Geometry check sheet. Reference: drawing and pictorial views, mm from the part's lowest x, y, z. Round coordinates to 2 decimals unless told otherwise and drop trailing zeros. Write each loop counter-clockwise with the first axis right and the second up, starting at its lowest first coordinate (ties: lowest second). Pieces come first, ordered by that corner, then holes. Notation, with made-up numbers: M -29,89 L 21,89 A13 cw 21,106 Z; hole C 32.5,72 d2. An arc over 180 degrees is marked long. One line per question, with ' | ' between items.
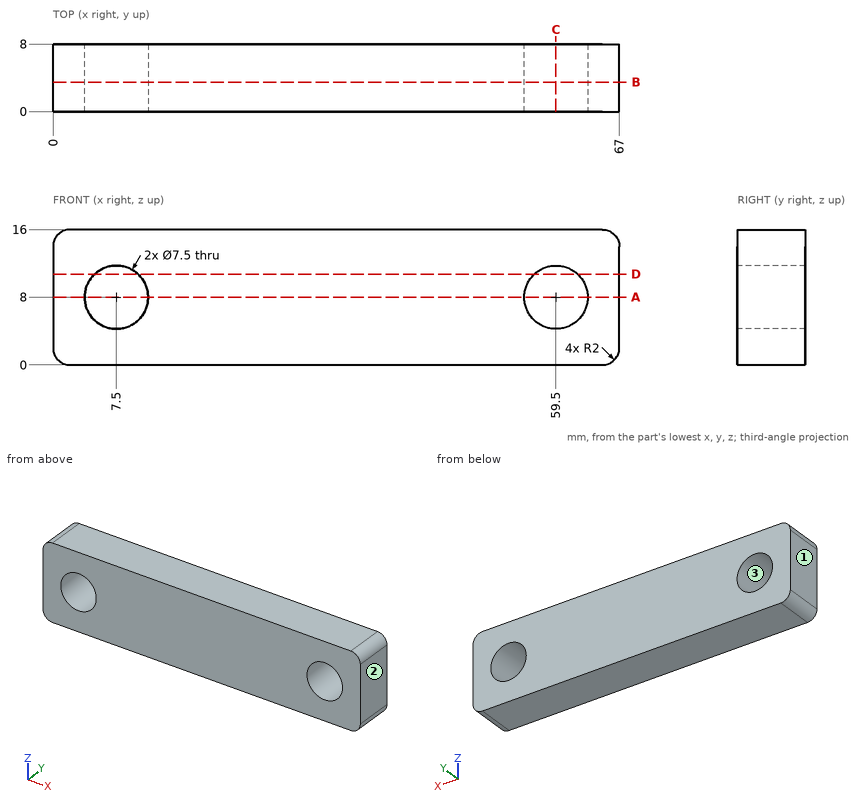
1. Section check C-C, the plane x = 59.5. Record the cut outline in (y, z).
Results:
outline: M 0,0 L 8,0 L 8,4.25 L 0,4.25 Z; M 0,11.75 L 8,11.75 L 8,16 L 0,16 Z
2. Section check D-D, the plane z = 10.75. Record the cut outline in (x, y), then the cut area to 3 significant figures.
Results:
outline: M 0,0 L 4.95,0 L 4.95,8 L 0,8 Z; M 10.05,0 L 56.95,0 L 56.95,8 L 10.05,8 Z; M 62.05,0 L 67,0 L 67,8 L 62.05,8 Z | area: 454 mm2
3. Section check B-B, the plane y = 3.5. Record the cut outline in (x, z).
Results:
outline: M 0,2 A2 ccw 2,0 L 65,0 A2 ccw 67,2 L 67,14 A2 ccw 65,16 L 2,16 A2 ccw 0,14 Z; hole C 7.5,8 d7.5; hole C 59.5,8 d7.5
4. Mould release check, pull along X, two halves, no side actions. Record for the marked faces 1, 2 and 3: pulls with the +X half, pulls with the -X half, needs draft (parallel to the pull), parting line crosses it, or undercut.
Results:
face 1: pulls with the -X half | face 2: pulls with the +X half | face 3: undercut
5. Thickness scan on line 1 (X direction, y = 4.25, z = 9.5); line 2 (Z direction, x = 7.5, y = 4.75); line 3 (X direction, y = 0.75, z = 6). Record the ranges inside material, lowest first.
Results:
line 1: x = 0 to 4.06, 10.94 to 56.06, 62.94 to 67 | line 2: z = 0 to 4.25, 11.75 to 16 | line 3: x = 0 to 4.33, 10.67 to 56.33, 62.67 to 67
6. Section check A-A, the plane z = 8. Record the cut outline in (x, y).
Results:
outline: M 0,0 L 3.75,0 L 3.75,8 L 0,8 Z; M 11.25,0 L 55.75,0 L 55.75,8 L 11.25,8 Z; M 63.25,0 L 67,0 L 67,8 L 63.25,8 Z
